```python
from build123d import *

# Parameters (mm, degrees)
SKETCH_R        = 9
SKETCH_R_2      = 1.6
PAD_DEPTH       = 3
SKETCH001_R     = 7.5
SKETCH001_R_2   = 5.2
PAD001_DEPTH    = 16
SKETCH002_W     = 19
SKETCH002_H     = 19
PAD002_DEPTH    = 3
SKETCH003_R     = 1.6
POCKET_DEPTH    = 3.001
SKETCH004_W     = 11
SKETCH004_H     = 8
PAD003_DEPTH    = 3
SKETCH005_R     = 1.6
POCKET001_DEPTH = 3.001
SKETCH007_R     = 5.2
SKETCH007_R_2   = 1.6
PAD004_DEPTH    = 4
SKETCH008_R     = 5.2
POCKET002_DEPTH = 4
CHAMFER_SIZE    = 1
FILLET_R        = 3.5


with BuildPart() as part:
    # Sketch → Pad (new body)
    with BuildSketch(Plane.XY):
        Circle(SKETCH_R)
        Circle(SKETCH_R_2, mode=Mode.SUBTRACT)
    extrude(amount=PAD_DEPTH)

    # Sketch001 (on Face4 of Pad) → Pad001 (join)
    with BuildSketch(Plane.XY.offset(3)):
        Circle(SKETCH001_R)
        Circle(SKETCH001_R_2, mode=Mode.SUBTRACT)
    extrude(amount=PAD001_DEPTH)

    # Sketch002 (on Face2 of Pad001) → Pad002 (join)
    with BuildSketch(Plane(origin=(0, 0, 0), x_dir=(1, 0, 0), z_dir=(0, 0, -1))):
        with Locations((-4.5, -4.5)):
            Rectangle(SKETCH002_W, SKETCH002_H)
    extrude(amount=-PAD002_DEPTH)

    # Sketch003 (on Face10 of Pad002) → Pocket (cut, through all)
    with BuildSketch(Plane.XY.offset(3)):
        Circle(SKETCH003_R)
    extrude(amount=-POCKET_DEPTH, mode=Mode.SUBTRACT)

    # Sketch004 (on Face16 of Pocket) → Pad003 (join)
    with BuildSketch(Plane.XY.offset(3)):
        with Locations((10.5, 0)):
            Rectangle(SKETCH004_W, SKETCH004_H)
    extrude(amount=-PAD003_DEPTH)

    # Sketch005 → Pocket001 (cut, through all)
    with BuildSketch(Plane.XY.offset(3)):
        with Locations((0, 10)):
            Circle(SKETCH005_R)
        with Locations((-10, 0)):
            Circle(SKETCH005_R)
        with Locations((10, 0)):
            Circle(SKETCH005_R)
    extrude(amount=-POCKET001_DEPTH, mode=Mode.SUBTRACT)

    # Sketch007 → Pad004 (join)
    with BuildSketch(Plane.XY.offset(3)):
        Circle(SKETCH007_R)
        Circle(SKETCH007_R_2, mode=Mode.SUBTRACT)
    extrude(amount=PAD004_DEPTH)

    # Sketch008 (on Face3 of Pad004) → Pocket002 (cut)
    with BuildSketch(Plane(origin=(0, 0, 0), x_dir=(1, 0, 0), z_dir=(0, 0, -1))):
        Circle(SKETCH008_R)
    extrude(amount=-POCKET002_DEPTH, mode=Mode.SUBTRACT)

    # Chamfer
    chamfer_edges = [part.edges().sort_by_distance(p)[0] for p in [
        (-5.2, 0, 19),
    ]]
    chamfer(chamfer_edges, length=CHAMFER_SIZE)

    # Fillet
    fillet_edges = [part.edges().sort_by_distance(p)[0] for p in [
        (5, 14, 1.5),
        (16, 4, 1.5),
        (-14, 14, 1.5),
        (-14, -5, 1.5),
        (16, -4, 1.5),
    ]]
    fillet(fillet_edges, radius=FILLET_R)


solid = part.part
```
Part model, mm, in its own coordinate system. A direction names the side the tool comes from. Give positions to 0.01 mm unless a question says otherwise; leave off trailing zeros. Write each loop counter-clockwise with the first axis right and the second up, starting at its lowest first coordinate (ties: lowest second). Pieces come first, ordered by that corner, then holes. Notation, with made-up numbers: M 19,13 L 55,13 A25 cw 55,38 Z; hole C 33,41.5 d7. An arc over 180 degrees is marked long. Use CSV: the item, a comma, the result in double quotes.
Item 1: Slice it at D-D on y = 10. Write the cut outline in (x, z), plus the area to 3 significant figures.
Taken from the geometry:
outline,"M -14,0 L -1.6,0 L -1.6,3 L -14,3 Z; M 1.6,0 L 5,0 L 5,3 L 1.6,3 Z"
area,"47.4 mm²"
Item 2: Slice it at A-A on x = 10. Write the cut outline in (y, z).
Taken from the geometry:
outline,"M -4,0 L -1.6,0 L -1.6,3 L -4,3 Z; M 1.6,0 L 4,0 L 4,3 L 1.6,3 Z"
Item 3: Slice it at B-B on x = 0. Write the cut outline in (y, z), plus the area to 3 significant figures.
Taken from the geometry:
outline,"M -9,0 L -5.2,0 L -5.2,4 L -1.6,4 L -1.6,7 L -5.2,7 L -5.2,18 L -6.2,19 L -7.5,19 L -7.5,3 L -9,3 Z; M 1.6,4 L 5.2,4 L 5.2,0 L 8.4,0 L 8.4,3 L 7.5,3 L 7.5,19 L 6.2,19 L 5.2,18 L 5.2,7 L 1.6,7 Z; M 11.6,0 L 14,0 L 14,3 L 11.6,3 Z"
area,"122 mm²"
Item 4: Slice it at C-C on y = 0. State how many separate pieces and enclosed holes the cut face has, plus the area to 3 significant figures.
Taken from the geometry:
separate pieces,"4"
enclosed holes,"0"
area,"134 mm²"
Item 5: Drill centre lines: probe 1 along Y at (x, z) = (0, 1.4); probe 2 along Y at (x, z) = (-10, 0.6); probe 3 along Y at (x, z) = (0, 9.5). Where is each one in solid material? Low to high.
Taken from the geometry:
probe 1,"y = -9 to -5.2, 5.2 to 8.4, 11.6 to 14"
probe 2,"y = -5 to -1.6, 1.6 to 14"
probe 3,"y = -7.5 to -5.2, 5.2 to 7.5"
Item 6: Pin check, flat tips, straight feed: P1, Ø8, axis at y = -1.5, z = 9, coming from the +X side; P2, Ø8.5, axis at x = -1, y = 0, coming from the +Z side; P3, Ø8.5, axis at x = 0, y = 0, coming from the +Z side. Stop position of each tip, or through.
Taken from the geometry:
P1,"stops at x = 7.5"
P2,"stops at z = 18.05"
P3,"stops at z = 7"
Item 7: Pull direction Y, two halves, no side cores. Call faces 4 (the face through (15, -2.95, 1.48)), 5 (the face through (6.78, 5.92, 1.48)), 6 (the face through (2, 0, 4)): +Y half, -Y half, draft (parallel to the pull), parting line (faces both ways), or undercut.
Taken from the geometry:
face 4,"-Y half"
face 5,"+Y half"
face 6,"undercut"
Item 8: Which spindle directions (+Z, -Z, +X, -X, +Y, -Y) get a long thin tool onto all of the face, cutting with end or side? Do faces 1 (the face through (5, 9, 1)), 2 (the face through (-7.493, 0.33, 10.888)), 3 (the face through (8.4, 0.07, 1.52)). Say none if no direction does.
Taken from the geometry:
face 1,"+Z, -Z, +X, +Y"
face 2,"+Z"
face 3,"+Z, -Z"
